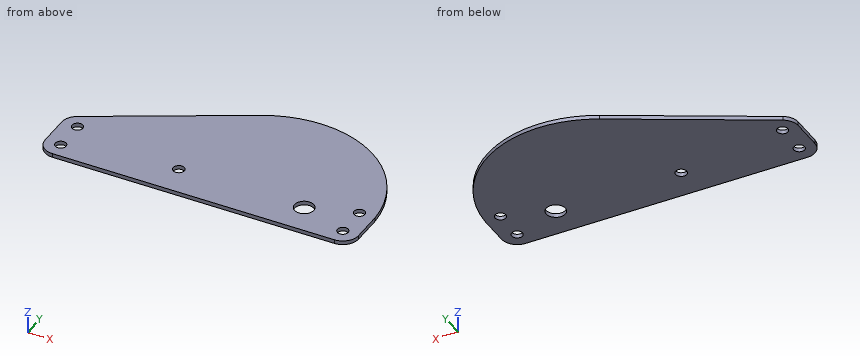
Autodesk Inventor part; units mm, degrees
ref_plane "YZ Plane" through (0, 0, 0) normal (1, 0, 0) x (0, 1, 0)
ref_plane "XZ Plane" through (0, 0, 0) normal (0, 1, 0) x (-1, 0, 0)
ref_plane "XY Plane" through (0, 0, 0) normal (0, 0, 1) x (1, 0, 0)
sketch "main" plane through (0, 0, 0) normal (0, 0, 1) x (1, 0, 0)
  circle A0 centre (50.5981, -28.4488) radius 2.1844
  line L0 (-66.7437, -10.1747) -> (-9.1578, 21.251)
  line L1 (50.5981, -34.7988) -> (-63.7019, -34.7988)
  circle A1 centre (50.5981, -15.7488) radius 2.1844
  arc A2 (50.5981, -34.7988) -> (56.9481, -28.4488) centre (50.5981, -28.4488) ccw
  line L2 (56.9481, -28.4488) -> (56.9481, -15.7488)
  arc A3 (56.9481, -15.7488) -> (56.9038, -14.9999) centre (50.5981, -15.7488) ccw
  arc A4 (56.9481, -15.7488) -> (-9.1578, 21.251) centre (12.2713, -18.0166) ccw
  circle A5 centre (31.5481, -22.0988) radius 3.9
  circle A6 centre (-19.2519, -22.0988) radius 2.2479
  circle A7 centre (-63.7019, -28.4488) radius 2.1844
  circle A8 centre (-63.7019, -15.7488) radius 2.1844
  arc A9 (-66.7437, -10.1747) -> (-70.0519, -15.7488) centre (-63.7019, -15.7488) ccw
  line L3 (-70.0519, -28.4488) -> (-70.0519, -15.7488)
  arc A10 (-70.0519, -28.4488) -> (-63.7019, -34.7988) centre (-63.7019, -28.4488) ccw
  point P0 (-3.3794, -19.3684)
  dimension "d0" = 7.8
  dimension "d1" = 4.4958
sketch "Sketch1" plane through (0, 0, 0) normal (0, 0, 1) x (1, 0, 0)
  circle A0 centre (0, 0) radius 2.1844
  line L0 (-117.3419, 18.274) -> (-59.7559, 49.6998)
  line L1 (0, -6.35) -> (-114.3, -6.35)
  circle A1 centre (0, 12.7) radius 2.1844
  arc A2 (0, -6.35) -> (6.35, 0) centre (0, 0) ccw
  line L2 (6.35, 0) -> (6.35, 12.7)
  arc A3 (6.35, 12.7) -> (6.3057, 13.4489) centre (0, 12.7) ccw
  arc A4 (6.35, 12.7) -> (-59.7559, 49.6998) centre (-38.3268, 10.4321) ccw
  circle A5 centre (-19.05, 6.35) radius 3.9
  circle A6 centre (-69.85, 6.35) radius 2.2479
  circle A7 centre (-114.3, 0) radius 2.1844
  circle A8 centre (-114.3, 12.7) radius 2.1844
  arc A9 (-117.3419, 18.274) -> (-120.65, 12.7) centre (-114.3, 12.7) ccw
  line L3 (-120.65, 0) -> (-120.65, 12.7)
  arc A10 (-120.65, 0) -> (-114.3, -6.35) centre (-114.3, 0) ccw
extrude "Extrusion1" add sketch "Sketch1" along normal blind 1.5875 contours L0 A4 L2 A2 L1 A10 L3 A9
properties part number "intake_sled" material "Acetal Resin, White"
Verification items for the finished model (mm, model axes). Give positions to 0.01 mm unless a question says otherwise; leave off trailing zeros. Order: outer loops, then holes, each group sorted by start corner. A loop starts at its lowest first (then second) coordinate and runs counter-clockwise, first axis right, second up. Notation, with made-up numbers: (61, 37.5) - (83, 37.5) arc R18 ccw to (83, 70.5) - close; hole circle Ø5 at (68, -7). An arc over 180 degrees is marked (long way). Answer as CSV lines item,"result". Start each with the question number.
Item 1: Material ranges on L1, parallel to Y at x = -114.3, z = 0.5; L2, parallel to Y at x = 0, z = 0.8; L3, parallel to Y at x = -69.85, z = 1.3, recorded low to high.
Item 2: Gauge pin test, flat ends, axial feed: pin 1 (2.5 mm diameter, centred on x = 0, y = 0, fed in from -Z); pin 2 (6 mm diameter, centred on x = -70, y = 45, fed in from -Z). Record the tip position at first contact, or that the pin passes through.
Item 3: Section check B-B, the plane y = 6.35. Record the boundary of the cut face in (x, z).
Item 4: Section check D-D, the plane y = 25. Record the boundary of the cut face in (x, z).
Item 5: Section check C-C, the plane x = -69.85. Record the boundary of the cut face in (y, z).
Item 6: Section check A-A, the plane z = 1.1. Record the boundary of the cut face in (x, y), plus the area to 3 significant figures.
Filled in:
1,L1,"-6.35 to -2.18, 2.18 to 10.52, 14.88 to 19.93"
1,L2,"-6.35 to -2.18, 2.18 to 10.52, 14.88 to 33.5"
1,L3,"-6.35 to 4.1, 8.6 to 44.19"
2,pin 1,"through"
2,pin 2,"z = 0"
3,outline,"(-120.65, 0) - (-72.1, 0) - (-72.1, 1.59) - (-120.65, 1.59) - close; (-67.6, 0) - (-22.95, 0) - (-22.95, 1.59) - (-67.6, 1.59) - close; (-15.15, 0) - (6.35, 0) - (6.35, 1.59) - (-15.15, 1.59) - close"
4,outline,"(-105.02, 0) - (3.97, 0) - (3.97, 1.59) - (-105.02, 1.59) - close"
5,outline,"(-6.35, 0) - (4.1, 0) - (4.1, 1.59) - (-6.35, 1.59) - close; (8.6, 0) - (44.19, 0) - (44.19, 1.59) - (8.6, 1.59) - close"
6,outline,"(-120.65, 0) arc R6.35 ccw to (-114.3, -6.35) - (0, -6.35) arc R6.35 ccw to (6.35, 0) - (6.35, 12.7) arc R44.73 ccw to (-59.76, 49.7) - (-117.34, 18.27) arc R6.35 ccw to (-120.65, 12.7) - close; hole circle Ø4.37 at (-114.3, 0); hole circle Ø4.37 at (-114.3, 12.7); hole circle Ø4.5 at (-69.85, 6.35); hole circle Ø7.8 at (-19.05, 6.35); hole circle Ø4.37 at (0, 0); hole circle Ø4.37 at (0, 12.7)"
6,area,"5,860 mm^2"
